from build123d import *

# Parameters (mm, degrees)
SKETCH_1_R      = 1.6
SKETCH_1_R_2    = 4
EXTRUDE_1_DEPTH = 3


with BuildPart() as part:
    # Sketch 1 → 填料-伸長1 (new body)
    with BuildSketch(Plane.XY):
        with BuildLine():
            Line((-5.221972445, 17.513309351), (-10.996349884, -4.724410549))
            Line((-10.996349884, -4.724410549), (-10.996349884, -16.06664646))
            ThreePointArc((-10.996349884, -16.06664646), (-0.137806793, -27.349136752), (10.99999726, -16.342235911))
            Line((10.99999726, -16.342235911), (10.99999726, -5))
            Line((10.99999726, -5), (15, -5))
            ThreePointArc((15, -5), (22.071067812, -2.071067812), (25, 5))
            Line((25, 5), (25, 15))
            ThreePointArc((25, 15), (22.071067812, 22.071067812), (15, 25))
            Line((15, 25), (4.4570397, 25))
            ThreePointArc((4.4570397, 25), (-1.661248724, 22.909901817), (-5.221972445, 17.513309351))
        make_face()
        with Locations((20, 20)):
            Circle(SKETCH_1_R, mode=Mode.SUBTRACT)
        with Locations((0, 20)):
            Circle(SKETCH_1_R, mode=Mode.SUBTRACT)
        Circle(SKETCH_1_R, mode=Mode.SUBTRACT)
        with Locations((20, 0)):
            Circle(SKETCH_1_R, mode=Mode.SUBTRACT)
        with Locations((0, -16.35)):
            Circle(SKETCH_1_R_2, mode=Mode.SUBTRACT)
        with Locations((8.5, -16.35)):
            Circle(SKETCH_1_R, mode=Mode.SUBTRACT)
        with Locations((6.01040764, -22.36040764)):
            Circle(SKETCH_1_R, mode=Mode.SUBTRACT)
        with Locations((0, -24.85)):
            Circle(SKETCH_1_R, mode=Mode.SUBTRACT)
        with Locations((-6.01040764, -22.36040764)):
            Circle(SKETCH_1_R, mode=Mode.SUBTRACT)
        with Locations((-8.5, -16.35)):
            Circle(SKETCH_1_R, mode=Mode.SUBTRACT)
        with Locations((-6.01040764, -10.33959236)):
            Circle(SKETCH_1_R, mode=Mode.SUBTRACT)
        with Locations((0, -7.85)):
            Circle(SKETCH_1_R, mode=Mode.SUBTRACT)
        with Locations((6.01040764, -10.33959236)):
            Circle(SKETCH_1_R, mode=Mode.SUBTRACT)
    extrude(amount=EXTRUDE_1_DEPTH)


solid = part.part
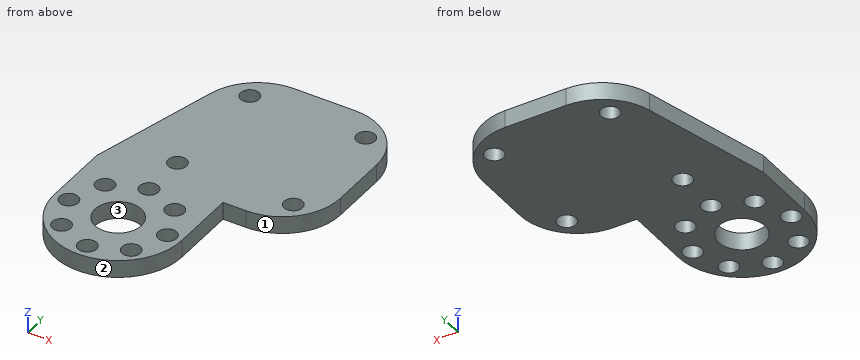
The listing builds one solid part. Answer for the finished solid, in the listing's coordinates (mm). Face numbers are marked on the shaded views. Give positions to 0.01 mm unless a question says otherwise; leave off trailing zeros. Write each loop counter-clockwise with the first axis right and the second up, starting at its lowest first coordinate (ties: lowest second). Pieces come first, ordered by that corner, then holes. Notation, with made-up numbers: (72.25, 73.25) -> (96.25, 73.25) arc R13 ccw to (96.25, 81.25) -> close; hole circle Ø3 at (70.25, 1). An arc over 180 degrees is marked (long way). One line per question, with ' | ' between items. Start each with the question number.
1. Section D-D (x = 5.5) is taken. Determine the outline of the cut face in (y, z).
2. Given pin 1 Ø3.5 at (x, y) = (8.5, -16.35) entering from +Z; pin 2 Ø1.5 at (x, z) = (-3, 2.5) entering from +Y, each flat-ended and moving along its own axis, determine where each tip first touches the part or whether it passes through.
3. Find the intervals of material crossed by probe 1 along Y at (x, z) = (0, 1.1); probe 2 along X at (y, z) = (-16.5, 2.1); probe 3 along X at (y, z) = (-23.5, 0.5), in increasing order.
4. Section B-B (x = -3) is taken. Determine the outline of the cut face in (y, z).
5. Section C-C (y = 19) is taken. Determine the outline of the cut face in (x, z).
6. Section A-A (y = -7.85) is taken. Determine the outline of the cut face in (x, z).
7. For a pull along X with two mould halves and no side action, classify the marked faces 1, 2 and 3 as pulls with the +X half, pulls with the -X half, needs draft (parallel to the pull), parting line crosses it, or undercut.
Response values:
1) outline: (-25.88, 0) -> (-23.88, 0) -> (-23.88, 3) -> (-25.88, 3) -> close; (-20.84, 0) -> (-11.86, 0) -> (-11.86, 3) -> (-20.84, 3) -> close; (-8.82, 0) -> (25, 0) -> (25, 3) -> (-8.82, 3) -> close
2) pin 1: z = 3 | pin 2: y = 22.42
3) probe 1: -27.35 to -26.45, -23.25 to -20.35, -12.35 to -9.45, -6.25 to -1.6, 1.6 to 18.4, 21.6 to 23.95 | probe 2: -11 to -10.09, -6.91 to -4, 4 to 6.91, 10.09 to 11 | probe 3: -8.36 to -7.13, -4.89 to -0.86, 0.86 to 4.89, 7.13 to 8.36
4) outline: (-26.93, 0) -> (-19, 0) -> (-19, 3) -> (-26.93, 3) -> close; (-13.7, 0) -> (21.66, 0) -> (21.66, 3) -> (-13.7, 3) -> close
5) outline: (-4.71, 0) -> (-1.25, 0) -> (-1.25, 3) -> (-4.71, 3) -> close; (1.25, 0) -> (18.75, 0) -> (18.75, 3) -> (1.25, 3) -> close; (21.25, 0) -> (24.17, 0) -> (24.17, 3) -> (21.25, 3) -> close
6) outline: (-11, 0) -> (-1.6, 0) -> (-1.6, 3) -> (-11, 3) -> close; (1.6, 0) -> (11, 0) -> (11, 3) -> (1.6, 3) -> close
7) face 1: pulls with the +X half | face 2: parting line crosses it | face 3: undercut
